```python
from build123d import *

# Parameters (mm, degrees)
ESQUISSE1_W             = 45
ESQUISSE1_H             = 6
BOSS_EXTRU_1_DEPTH      = 10
BOSS_EXTRU_1_2_DEPTH    = 10
ESQUISSE2_W             = 75
ESQUISSE2_H             = 50
ESQUISSE2_R             = 2.5
BOSS_EXTRU_2_DEPTH      = 5
ENL_V_MAT_EXTRU_1_REACH = 55.278
ESQUISSE3_R             = 2.5


with BuildPart() as part:
    # Esquisse1 → Boss.-Extru.1 (new body)
    with BuildSketch(Plane.XY):
        with Locations((0, 8.5)):
            Rectangle(ESQUISSE1_W, ESQUISSE1_H)
    extrude(amount=BOSS_EXTRU_1_DEPTH)



with BuildPart() as body_2:
    # Esquisse1 → Boss.-Extru.1 2 (new body)
    with BuildSketch(Plane.XY):
        with Locations((0, -8.5)):
            Rectangle(ESQUISSE1_W, ESQUISSE1_H)
    extrude(amount=BOSS_EXTRU_1_2_DEPTH)


with BuildPart() as part_1:
    add(part.part)

    add(body_2.part)  # Boss.-Extru.2 merges body 2
    # Esquisse2 → Boss.-Extru.2 (add)
    with BuildSketch(Plane(origin=(0, 0, 0), x_dir=(-1, 0, 0), z_dir=(0, 0, -1))):
        Rectangle(ESQUISSE2_W, ESQUISSE2_H)
        with Locations((32.5, 20)):
            Circle(ESQUISSE2_R, mode=Mode.SUBTRACT)
        with Locations(Location((-32.5, 20, 0), (0, 0, 180))):
            Circle(ESQUISSE2_R, mode=Mode.SUBTRACT)
        with Locations((-32.5, -20)):
            Circle(ESQUISSE2_R, mode=Mode.SUBTRACT)
        with Locations(Location((32.5, -20, 0), (0, 0, 180))):
            Circle(ESQUISSE2_R, mode=Mode.SUBTRACT)
    extrude(amount=BOSS_EXTRU_2_DEPTH)

    # Enlèv. mat.-Extru.1: up to this face of the body (flat: up to its plane)
    enl_v_mat_extru_1_end = Plane(part_1.part.faces().sort_by_distance((0, 11.5, 5))[0])
    # Esquisse3 → Enlèv. mat.-Extru.1 (cut, up to the picked face)
    with BuildSketch(Plane.XZ.offset(11.5), mode=Mode.PRIVATE) as enl_v_mat_extru_1_sk1:
        with Locations(Location((-5, 5.0183964, 0), (0, 0, 270))):
            Circle(ESQUISSE3_R)
    enl_v_mat_extru_1_tool1 = split(extrude(enl_v_mat_extru_1_sk1.sketch, amount=-ENL_V_MAT_EXTRU_1_REACH, mode=Mode.PRIVATE), bisect_by=enl_v_mat_extru_1_end, keep=Keep.BOTH, mode=Mode.PRIVATE)
    # Esquisse3 → Enlèv. mat.-Extru.1 (cut, up to the picked face)
    with BuildSketch(Plane.XZ.offset(11.5), mode=Mode.PRIVATE) as enl_v_mat_extru_1_sk2:
        with Locations(Location((5, 5.0183964, 0), (0, 0, 270))):
            Circle(ESQUISSE3_R)
    enl_v_mat_extru_1_tool2 = split(extrude(enl_v_mat_extru_1_sk2.sketch, amount=-ENL_V_MAT_EXTRU_1_REACH, mode=Mode.PRIVATE), bisect_by=enl_v_mat_extru_1_end, keep=Keep.BOTH, mode=Mode.PRIVATE)
    # Esquisse3 → Enlèv. mat.-Extru.1 (cut, up to the picked face)
    with BuildSketch(Plane.XZ.offset(11.5), mode=Mode.PRIVATE) as enl_v_mat_extru_1_sk3:
        with Locations(Location((15, 5.0183964, 0), (0, 0, 270))):
            Circle(ESQUISSE3_R)
    enl_v_mat_extru_1_tool3 = split(extrude(enl_v_mat_extru_1_sk3.sketch, amount=-ENL_V_MAT_EXTRU_1_REACH, mode=Mode.PRIVATE), bisect_by=enl_v_mat_extru_1_end, keep=Keep.BOTH, mode=Mode.PRIVATE)
    # Esquisse3 → Enlèv. mat.-Extru.1 (cut, up to the picked face)
    with BuildSketch(Plane.XZ.offset(11.5), mode=Mode.PRIVATE) as enl_v_mat_extru_1_sk4:
        with Locations(Location((-15, 5.0183964, 0), (0, 0, 270))):
            Circle(ESQUISSE3_R)
    enl_v_mat_extru_1_tool4 = split(extrude(enl_v_mat_extru_1_sk4.sketch, amount=-ENL_V_MAT_EXTRU_1_REACH, mode=Mode.PRIVATE), bisect_by=enl_v_mat_extru_1_end, keep=Keep.BOTH, mode=Mode.PRIVATE)
    add(enl_v_mat_extru_1_tool1.solids().sort_by(Axis((-5, -11.5, 5.018396), (0, 1, 0)))[0], mode=Mode.SUBTRACT)
    add(enl_v_mat_extru_1_tool2.solids().sort_by(Axis((5, -11.5, 5.018396), (0, 1, 0)))[0], mode=Mode.SUBTRACT)
    add(enl_v_mat_extru_1_tool3.solids().sort_by(Axis((15, -11.5, 5.018396), (0, 1, 0)))[0], mode=Mode.SUBTRACT)
    add(enl_v_mat_extru_1_tool4.solids().sort_by(Axis((-15, -11.5, 5.018396), (0, 1, 0)))[0], mode=Mode.SUBTRACT)


solid = part_1.part
```
The model under review builds one solid part; all positions refer to its coordinate system, in mm. A direction names the side the tool comes from. Coordinates: 2 decimals unless noted, no trailing zeros. Order: outer loops, then holes, each group sorted by start corner. A loop starts at its lowest first (then second) coordinate and runs counter-clockwise, first axis right, second up. Notation, with made-up numbers: (26, -10) -> (75, -10) arc R9 ccw to (75, 7) -> close; hole circle Ø11 at (80, 74.25). An arc over 180 degrees is marked (long way). Answer in a Markdown table with one row per item. Add a question column.
Item 1: Clearance check with flat-ended pins moving along their axes: pin 1 (1 mm diameter, centred on y = -9.5, z = 5.5, fed in from +X); pin 2 (3 mm diameter, centred on x = 3, z = 5, fed in from +Y); pin 3 (8 mm diameter, centred on x = -10, z = 7.5, fed in from -Y). State where each tip first meets the part, or that it passes through.
Item 2: We need section A-A on z = 8.5. Write out the cut boundary in (x, y), plus the area to 3 significant figures.
Item 3: We need section D-D on x = 32.5. Write out the cut boundary in (y, z), plus the area to 3 significant figures.
Item 4: We need section B-B on x = -5. Write out the cut boundary in (y, z), plus the area to 3 significant figures.
Item 5: To check wall thickness, follow probe 1 along X at (y, z) = (-9, 5.25); probe 2 along X at (y, z) = (6, 3.75); probe 3 along Y at (x, z) = (-5.5, 2.25). State the ranges of each line that lie inside material, in increasing order.
Item 6: Mouldability with a two-part tool opening along Z and no side actions: class faces 1 (the flat face through (1, 0, 0)), 2 (the cylindrical face through (-17.44, -8.54, 5.56)), 3 (the cylindrical face through (-17.44, 8.46, 5.56)), 4 (the flat face through (-37.5, 0, -2)) as +Z half, -Z half, draft (parallel to the pull), parting line (faces both ways), or undercut.
Item 7: Machinability: for faces 5 (the flat face through (22.5, 8, 5)), 6 (the flat face through (0, -5.5, 5)), 7 (the flat face through (0, -11.5, 5)), which of the approach directions +Z, -Z, +X, -X, +Y, -Y give a long, thin tool a straight path to every point of the face, cutting with its end or side? Answer none if there is none.
Item 8: We need section C-C on y = 20. Write out the cut boundary in (x, z).
Final values:
| question | item | result |
|---|---|---|
| 1 | pin 1 | stops at x = 22.5 |
| 1 | pin 2 | stops at y = 11.5 |
| 1 | pin 3 | stops at y = -11.5 |
| 2 | outline | (-22.5, -11.5) -> (22.5, -11.5) -> (22.5, -5.5) -> (-22.5, -5.5) -> close; (-22.5, 5.5) -> (22.5, 5.5) -> (22.5, 11.5) -> (-22.5, 11.5) -> close |
| 2 | area | 540 mm2 |
| 3 | outline | (-25, -5) -> (-22.5, -5) -> (-22.5, 0) -> (-25, 0) -> close; (-17.5, -5) -> (17.5, -5) -> (17.5, 0) -> (-17.5, 0) -> close; (22.5, -5) -> (25, -5) -> (25, 0) -> (22.5, 0) -> close |
| 3 | area | 200 mm2 |
| 4 | outline | (-25, -5) -> (25, -5) -> (25, 0) -> (11.5, 0) -> (11.5, 2.52) -> (5.5, 2.52) -> (5.5, 0) -> (-5.5, 0) -> (-5.5, 2.52) -> (-11.5, 2.52) -> (-11.5, 0) -> (-25, 0) -> close; (-11.5, 7.52) -> (-5.5, 7.52) -> (-5.5, 10) -> (-11.5, 10) -> close; (5.5, 7.52) -> (11.5, 7.52) -> (11.5, 10) -> (5.5, 10) -> close |
| 4 | area | 310 mm2 |
| 5 | probe 1 | x = -22.5 to -17.49, -12.51 to -7.49, -2.51 to 2.51, 7.49 to 12.51, 17.49 to 22.5 |
| 5 | probe 2 | x = -22.5 to -17.15, -12.85 to -7.15, -2.85 to 2.85, 7.15 to 12.85, 17.15 to 22.5 |
| 5 | probe 3 | y = -11.5 to -5.5, 5.5 to 11.5 |
| 6 | face 1 | +Z half |
| 6 | face 2 | undercut |
| 6 | face 3 | undercut |
| 6 | face 4 | draft |
| 7 | face 5 | +Z, +X, +Y, -Y |
| 7 | face 6 | +Z, +X, -X |
| 7 | face 7 | +Z, +X, -X, -Y |
| 8 | outline | (-37.5, -5) -> (-35, -5) -> (-35, 0) -> (-37.5, 0) -> close; (-30, -5) -> (30, -5) -> (30, 0) -> (-30, 0) -> close; (35, -5) -> (37.5, -5) -> (37.5, 0) -> (35, 0) -> close |
